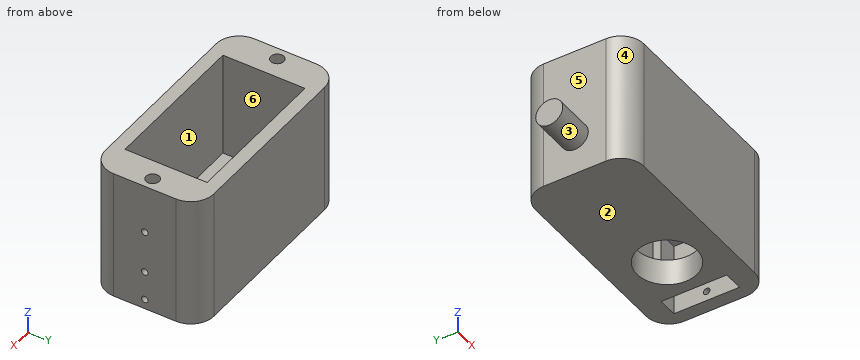
```python
from build123d import *

# Parameters (mm, degrees)
SKETCH1_W           = 33
SKETCH1_H           = 16.5
SKETCH1_W_2         = 23
SKETCH1_H_2         = 12.5
BOSS_EXTRUDE1_DEPTH = 16
SKETCH2_R           = 1
CUT_EXTRUDE1_DEPTH  = 4
SKETCH6_R           = 4.575
BOSS_EXTRUDE5_DEPTH = 4
SKETCH7_W           = 3
SKETCH7_H           = 10
CUT_EXTRUDE3_DEPTH  = 11
SKETCH9_R           = 0.5
CUT_EXTRUDE4_DEPTH  = 4
SKETCH10_R          = 2.06
BOSS_EXTRUDE6_DEPTH = 6
FILLET1_R           = 3.5


with BuildPart() as part:
    # Sketch1 → Boss-Extrude1 (new body)
    with BuildSketch(Plane.XY):
        Rectangle(SKETCH1_W, SKETCH1_H)
        Rectangle(SKETCH1_W_2, SKETCH1_H_2, mode=Mode.SUBTRACT)
    extrude(amount=BOSS_EXTRUDE1_DEPTH)

    # Sketch2 → Cut-Extrude1 (cut)
    with BuildSketch(Plane.XY.offset(16)):
        with Locations((-14.65, 0)):
            Circle(SKETCH2_R)
        with Locations(Location((14.65, 0, 0), (0, 0, 180))):
            Circle(SKETCH2_R)
    extrude(amount=-CUT_EXTRUDE1_DEPTH, mode=Mode.SUBTRACT)

    # Sketch6 → Boss-Extrude5 (add)
    with BuildSketch(Plane(origin=(0, 0, 0), x_dir=(-1, 0, 0), z_dir=(0, 0, -1))):
        Polygon((-11.5, 8.25), (16.5, 8.25), (16.5, -8.25), (-11.5, -8.25), (-16.5, -8.25), (-16.5, 8.25), align=None)
        with Locations((-5.175, 0)):
            Circle(SKETCH6_R, mode=Mode.SUBTRACT)
    extrude(amount=BOSS_EXTRUDE5_DEPTH)

    # Sketch7 → Cut-Extrude3 (cut)
    with BuildSketch(Plane(origin=(0, 0, -4), x_dir=(-1, 0, 0), z_dir=(0, 0, -1))):
        with Locations((-13, 0)):
            Rectangle(SKETCH7_W, SKETCH7_H)
    extrude(amount=-CUT_EXTRUDE3_DEPTH, mode=Mode.SUBTRACT)

    # Sketch9 → Cut-Extrude4 (cut)
    with BuildSketch(Plane(origin=(16.5, 0, 0), x_dir=(0, 0, -1), z_dir=(1, 0, 0))):
        with Locations((-2, 0)):
            Circle(SKETCH9_R)
        with Locations((2.5, 0)):
            Circle(SKETCH9_R)
        with Locations((-8.5, 0)):
            Circle(SKETCH9_R)
    extrude(amount=-CUT_EXTRUDE4_DEPTH, mode=Mode.SUBTRACT)

    # Sketch10 → Boss-Extrude6 (add)
    with BuildSketch(Plane.ZY.offset(16.5)):
        with Locations(Location((2, 0, 0), (0, 0, 180))):
            Circle(SKETCH10_R)
    extrude(amount=BOSS_EXTRUDE6_DEPTH)

    # Fillet1
    fillet1_edges = [part.edges().sort_by_distance(p)[0] for p in [
        (16.5, -8.25, 6),
        (-16.5, -8.25, 6),
        (-16.5, 8.25, 6),
        (16.5, 8.25, 6),
    ]]
    fillet(fillet1_edges, radius=FILLET1_R)


solid = part.part
```
Could you check a few things on this model? Use its own coordinates, in mm. Face numbers are marked on the shaded views. A direction names the side the tool comes from. Give positions to 0.01 mm unless a question says otherwise; leave off trailing zeros. Write each loop counter-clockwise with the first axis right and the second up, starting at its lowest first coordinate (ties: lowest second). Pieces come first, ordered by that corner, then holes. Notation, with made-up numbers: (88, 76) -> (135, 76) arc R28 ccw to (135, 99) -> close; hole circle Ø4 at (67.25, 89.5). An arc over 180 degrees is marked (long way). Write each question's results on one line, items separated by ' | '.
1. I want a section at D-D, the plane y = -5.5. Write out the boundary of the cut face in (x, z), then the cut area to 3 significant figures.
Check sheet entries:
outline: (-16.42, -4) -> (16.42, -4) -> (16.42, 16) -> (11.5, 16) -> (11.5, 0) -> (-11.5, 0) -> (-11.5, 16) -> (-16.42, 16) -> close | area: 289 mm²
2. If we mould it in two halves opening along Y, with no side actions, what happens to the marked faces 4, 5 and 6? For each: released by +Y, released by -Y, zero draft, split by the parting line, or undercut.
Check sheet entries:
face 4: released by -Y | face 5: zero draft | face 6: undercut
3. Will these pins go through, and if not, where does the flat tip stop? pin 1 Ø6 at (y, z) = (1.5, 9.5) entering from -X; pin 2 Ø4 at (x, y) = (-5, 2.5) entering from +Z; pin 3 Ø0.9 at (x, y) = (13.5, -2) entering from -Z.
Check sheet entries:
pin 1: stops at x = -16.5 | pin 2: stops at z = 0 | pin 3: stops at z = 7
4. I want a section at C-C, the plane x = 2.5. Write out the boundary of the cut face in (y, z), then the cut area to 3 significant figures.
Check sheet entries:
outline: (-8.25, -4) -> (-3.71, -4) -> (-3.71, 0) -> (-6.25, 0) -> (-6.25, 16) -> (-8.25, 16) -> close; (3.71, -4) -> (8.25, -4) -> (8.25, 16) -> (6.25, 16) -> (6.25, 0) -> (3.71, 0) -> close | area: 100 mm²
5. I want a section at B-B, the plane z = 12.75. Write out the boundary of the cut face in (x, y).
Check sheet entries:
outline: (-16.5, -4.75) arc R3.5 ccw to (-13, -8.25) -> (13, -8.25) arc R3.5 ccw to (16.5, -4.75) -> (16.5, 4.75) arc R3.5 ccw to (13, 8.25) -> (-13, 8.25) arc R3.5 ccw to (-16.5, 4.75) -> close; hole circle Ø2 at (-14.65, 0); hole (-11.5, -6.25) -> (11.5, -6.25) -> (11.5, 6.25) -> (-11.5, 6.25) -> close; hole circle Ø2 at (14.65, 0)
6. I need wall thicknesses on L1, parallel to X at y = -4, z = 1.25; L2, parallel to X at y = 1.5, z = 14.25; L3, parallel to X at y = -1.75, z = -2.5. Which ranges of each line are inside material? Lowest first, please.
Check sheet entries:
L1: x = -16.5 to -11.5, 14.5 to 16.5 | L2: x = -16.5 to -11.5, 11.5 to 16.5 | L3: x = -16.5 to 0.95, 9.4 to 11.5, 14.5 to 16.5
7. On a 3-axis mill with a long thin cutter (end or side, diameter ignored), from which of +Z, -Z, +X, -X, +Y, -Y can I reach the whole of each face in a straight line? I mean the marked faces 1, 2 and 3. Say none if no direction works.
Check sheet entries:
face 1: +Z | face 2: -Z, +X, -X, +Y, -Y | face 3: -X
8. I want a section at A-A, the plane z = 8.5. Write out the boundary of the cut face in (x, y), then the cut area to 3 significant figures.
Check sheet entries:
outline: (-16.5, -4.75) arc R3.5 ccw to (-13, -8.25) -> (13, -8.25) arc R3.5 ccw to (16.5, -4.75) -> (16.5, -0.5) -> (12.5, -0.5) -> (12.5, 0.5) -> (16.5, 0.5) -> (16.5, 4.75) arc R3.5 ccw to (13, 8.25) -> (-13, 8.25) arc R3.5 ccw to (-16.5, 4.75) -> close; hole (-11.5, -6.25) -> (11.5, -6.25) -> (11.5, 6.25) -> (-11.5, 6.25) -> close | area: 242 mm²
